from build123d import *

# Parameters (mm, degrees)
SKETCH1_W           = 4.721281475
SKETCH1_H           = 1.214825
BOSS_EXTRUDE1_DEPTH = 1.5
FILLET1_R           = 1
FILLET2_R           = 1
CUT_EXTRUDE1_DEPTH  = 2
LPATTERN1_COUNT     = 4
LPATTERN1_PITCH     = 0.75


with BuildPart() as part:
    # Sketch1 → Boss-Extrude1 (new body)
    with BuildSketch(Plane(origin=(0, 0, 0), x_dir=(1, 0, 0), z_dir=(0, 1, 0))):
        Polygon((-42.085271319, 4.006512849), (-41.335271319, 4.006512849), (-41.335271319, 15.221337849), (-42.085271319, 15.221337849), (-42.085271319, 10.221337849), (-42.085271319, 9.006512849), align=None)
        with Locations((-44.445912057, 9.613925349)):
            Rectangle(SKETCH1_W, SKETCH1_H)
    extrude(amount=BOSS_EXTRUDE1_DEPTH)

    # Fillet1
    fillet1_edges = [part.edges().sort_by_distance(p)[0] for p in [
        (-42.085271319, 0.75, -10.221337849),
    ]]
    fillet(fillet1_edges, radius=FILLET1_R)

    # Fillet2
    fillet2_edges = [part.edges().sort_by_distance(p)[0] for p in [
        (-42.085271319, 0.75, -9.006512849),
    ]]
    fillet(fillet2_edges, radius=FILLET2_R)

    # Sketch2 → Cut-Extrude1 (cut)
    with BuildSketch(Plane(origin=(0, 1.5, 0), x_dir=(1, 0, 0), z_dir=(0, 1, 0))):
        with BuildLine():
            ThreePointArc((-45.796552794, 10.221337849), (-46.046552794, 10.471337849), (-46.296552794, 10.221337849))
            Line((-46.296552794, 10.221337849), (-46.046552794, 10.221337849))
            Line((-46.046552794, 10.221337849), (-45.796552794, 10.221337849))
        make_face()
        with BuildLine():
            Line((-46.046552794, 10.221337849), (-46.296552794, 10.221337849))
            ThreePointArc((-46.296552794, 10.221337849), (-46.046552794, 9.971337849), (-45.796552794, 10.221337849))
            Line((-45.796552794, 10.221337849), (-46.046552794, 10.221337849))
        make_face()
    cut_extrude1 = extrude(amount=-CUT_EXTRUDE1_DEPTH, mode=Mode.SUBTRACT)

    # LPattern1: Cut-Extrude1 ×4
    with Locations(*[(i * LPATTERN1_PITCH, 0, 0) for i in range(1, LPATTERN1_COUNT)]):
        add(cut_extrude1, mode=Mode.SUBTRACT)


solid = part.part
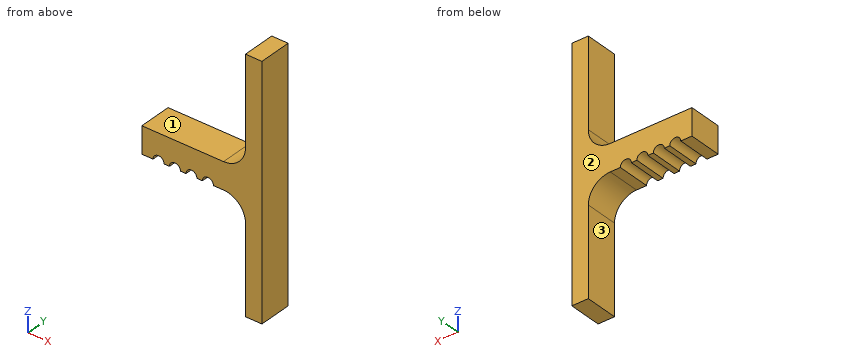
Geometry check sheet. Reference: the model listing, model coordinates, mm. Face numbers are marked on the shaded views. A direction names the side the tool comes from. Give positions to 0.01 mm unless a question says otherwise; leave off trailing zeros. Write each loop counter-clockwise with the first axis right and the second up, starting at its lowest first coordinate (ties: lowest second). Pieces come first, ordered by that corner, then holes.
1) Cross-section at A-A (y = 1.15). Record the boundary of the cut face in (x, z), plus the area to 3 significant figures.
Values follow:
outline: (-46.81, -10.22) - (-46.3, -10.22) arc R0.25 cw to (-45.8, -10.22) - (-45.55, -10.22) arc R0.25 cw to (-45.05, -10.22) - (-44.8, -10.22) arc R0.25 cw to (-44.3, -10.22) - (-44.05, -10.22) arc R0.25 cw to (-43.55, -10.22) - (-43.09, -10.22) arc R1 cw to (-42.09, -11.22) - (-42.09, -15.22) - (-41.34, -15.22) - (-41.34, -4.01) - (-42.09, -4.01) - (-42.09, -8.01) arc R1 cw to (-43.09, -9.01) - (-46.81, -9.01) - close
area: 14.2 mm2
2) Go/stop test with flat-tipped pins: pin 1 Ø1.5 at (x, z) = (-46, -9) entering from -Y; pin 2 Ø2 at (x, z) = (-45, -11.5) entering from -Y; pin 3 Ø0.8 at (x, y) = (-44, 1) entering from +Z. Record where each tip stops, or that it passes through.
Values follow:
pin 1: stops at y = 0
pin 2: passes through
pin 3: stops at z = -9.01
3) Set-up check for the marked faces 1, 2 and 3: record each of +Z, -Z, +X, -X, +Y, -Y from which the full face is reachable in a straight line by a thin tool's end or side.
Values follow:
face 1: +Z, -X, +Y, -Y
face 2: +Z, -Z, +X, -X, +Y
face 3: -Z, -X, +Y, -Y
4) Cross-section at C-C (z = -4.75). Record the boundary of the cut face in (x, y), plus the area to 4 significant figures.
Values follow:
outline: (-42.09, 0) - (-41.34, 0) - (-41.34, 1.5) - (-42.09, 1.5) - close
area: 1.125 mm2
5) Cross-section at B-B (x = -43.35). Record the boundary of the cut face in (y, z).
Values follow:
outline: (0, -10.22) - (1.5, -10.22) - (1.5, -9.01) - (0, -9.01) - close
6) Thickness scan on line 1 (Z direction, x = -43.2, y = 0.9); line 2 (X direction, y = 0.95, z = -11.5); line 3 (Z direction, x = -42.45, y = 1.35). Record the ranges inside material, lowest first.
Values follow:
line 1: z = -10.22 to -9.01
line 2: x = -42.09 to -41.34
line 3: z = -10.45 to -8.78
